Can you work these out from the drawing? Everything is in mm from the part's minimum corner. A direction names the side the tool comes from. Coordinates: 2 decimals unless noted, no trailing zeros. Use a Markdown table: item, result. Add a question column.
1) If I drill on L1, parallel to Y at x = 9, z = 7.75 (1 decimal); L2, parallel to X at y = 5.5, z = 5.25 (1 decimal); L3, parallel to Z at x = 7.25, y = 2.75 (1 decimal), over which ranges is the centre line in solid material (lowest first)? Write a range as [from, to].
2) Thinking about a two-plate mould opening in Z: for the marked faces 1, 2 and 3, which applies, +Z half, -Z half, draft (parallel to the pull), parting line (faces both ways), or undercut?
3) Which directions (+Z, -Z, +X, -X, +Y, -Y) give clear straight access to the entire face, cutting with the end or side of a thin tool? Please do the marked faces 4, 5 and 6.
4) Will these pins go through, and if not, where does the flat tip stop? pin 1 Ø3 at (y, z) = (5.5, 1.5) entering from +X (1 decimal); pin 2 Ø3.5 at (x, y) = (6, 2) entering from -Z; pin 3 Ø1 at (x, y) = (5.5, 4.5) entering from +Z; pin 4 Ø3 at (x, z) = (7.5, 5.5) entering from +Y (1 decimal).
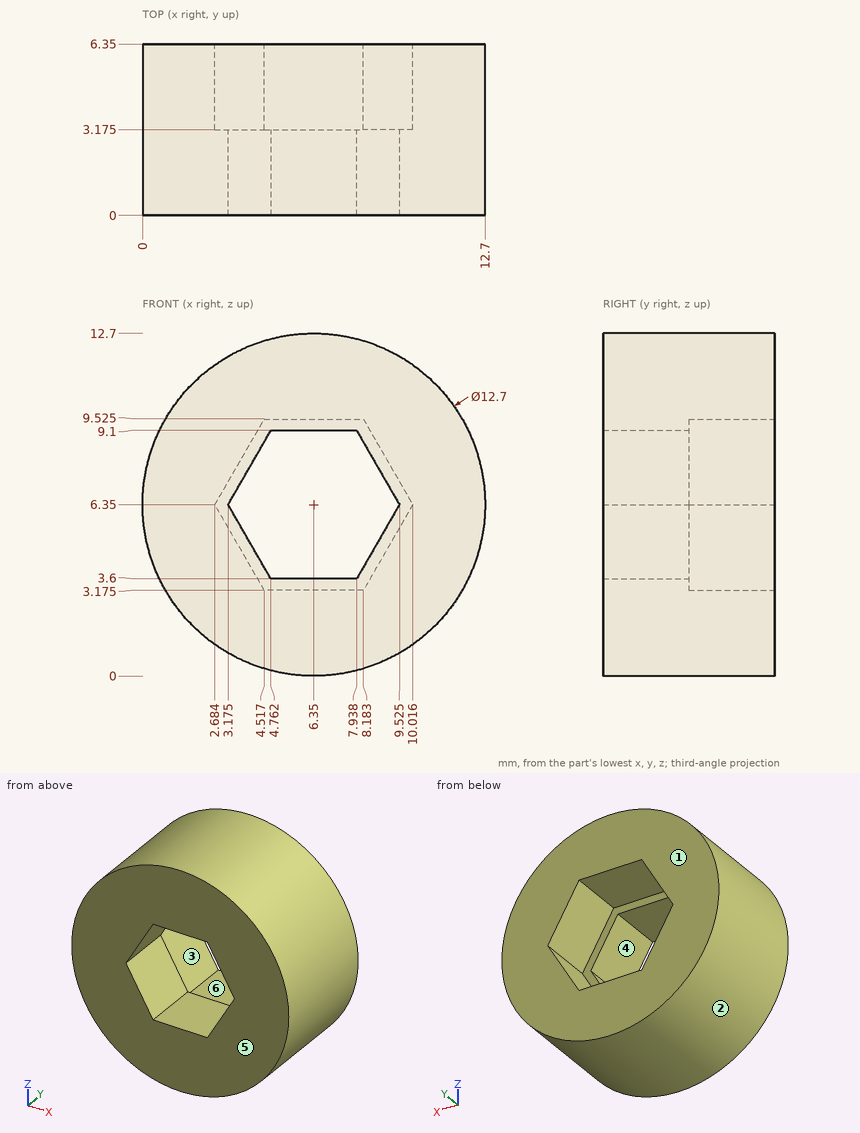
Answer sheet:
| question | item | result |
|---|---|---|
| 1 | L1 | [0, 3.2] |
| 1 | L2 | [0.1, 3.3], [9.4, 12.6] |
| 1 | L3 | [0.1, 3.6], [9.1, 12.6] |
| 2 | face 1 | draft |
| 2 | face 2 | parting line |
| 2 | face 3 | undercut |
| 3 | face 4 | +Y, -Y |
| 3 | face 5 | +Z, -Z, +X, -X, -Y |
| 3 | face 6 | +Y |
| 4 | pin 1 | x = 11.7 |
| 4 | pin 2 | z = 0 |
| 4 | pin 3 | z = 12.69 |
| 4 | pin 4 | y = 3.2 |
